from build123d import *

# Parameters (mm, degrees)
SKETCH1_R           = 1
BOSS_EXTRUDE1_DEPTH = 5
FILLET1_R           = 5
FILLET2_R           = 5
FILLET3_R           = 5
FILLET4_R           = 3


with BuildPart() as part:
    # Sketch1 → Boss-Extrude1 (new, symmetric)
    with BuildSketch(Plane(origin=(0, 0, 0), x_dir=(1, 0, 0), z_dir=(0, 1, 0))):
        Polygon((0, -60), (-14.281480067, -70), (-61.501480067, -70), (-99.58, -32.62), (-99.58, 0), (99.58, 0), (99.58, -32.62), (61.501480067, -70), (14.281480067, -70), align=None)
        with Locations(Location((96.58, -8.16, 0), (0, 0, 270))):
            Circle(SKETCH1_R, mode=Mode.SUBTRACT)
        with Locations(Location((96.58, -16.32, 0), (0, 0, 270))):
            Circle(SKETCH1_R, mode=Mode.SUBTRACT)
        with Locations(Location((96.58, -24.48, 0), (0, 0, 270))):
            Circle(SKETCH1_R, mode=Mode.SUBTRACT)
        with Locations(Location((-96.58, -24.48, 0), (0, 0, 90))):
            Circle(SKETCH1_R, mode=Mode.SUBTRACT)
        with Locations(Location((-96.58, -16.32, 0), (0, 0, 90))):
            Circle(SKETCH1_R, mode=Mode.SUBTRACT)
        with Locations(Location((-96.58, -8.16, 0), (0, 0, 90))):
            Circle(SKETCH1_R, mode=Mode.SUBTRACT)
    extrude(amount=BOSS_EXTRUDE1_DEPTH, both=True)

    # Fillet1
    fillet1_edges = [part.edges().sort_by_distance(p)[0] for p in [
        (-14.281480067, 0, 70),
        (14.281480067, 0, 70),
    ]]
    fillet(fillet1_edges, radius=FILLET1_R)

    # Fillet2
    fillet2_edges = [part.edges().sort_by_distance(p)[0] for p in [
        (-61.501480067, 0, 70),
        (61.501480067, 0, 70),
    ]]
    fillet(fillet2_edges, radius=FILLET2_R)

    # Fillet3
    fillet3_edges = [part.edges().sort_by_distance(p)[0] for p in [
        (-99.58, 0, 32.62),
        (99.58, 0, 32.62),
    ]]
    fillet(fillet3_edges, radius=FILLET3_R)

    # Fillet4
    fillet4_edges = [part.edges().sort_by_distance(p)[0] for p in [
        (-99.58, 0, 0),
        (99.58, 0, 0),
    ]]
    fillet(fillet4_edges, radius=FILLET4_R)

    # Fillet5
    # a fillet whose section is not a circle: 8 mm, written as the material it adds along each edge
    with BuildSketch(Plane(origin=(0, -5, 60), x_dir=(-0.8191520442889911, 0, 0.5735764363510473), z_dir=(0, 1, 0))) as fillet5_piece_1:
        with BuildLine():
            Bezier((5.601660306, 0), (0, 0), (-1.915880661, 5.263838853), weights=[1, 1, 1])
            Line((-1.915880661, 5.263838853), (0, 0))
            Line((0, 0), (5.601660306, 0))
        make_face()
    extrude(amount=10)


solid = part.part
Read the model definition and answer for the solid it produces. Units are mm, in the model's axes. Round coordinates to 2 decimals unless told otherwise and drop trailing zeros. Write each loop counter-clockwise with the first axis right and the second up, starting at its lowest first coordinate (ties: lowest second). Pieces come first, ordered by that corner, then holes.
Q1. Find section D-D on z = 54. Determine the outline of the cut face in (x, y), and give its area (3 significant figures).
Values:
outline: (-77.8, -5) - (77.8, -5) - (77.8, 5) - (-77.8, 5) - close
area: 1,560 mm2
Q2. The mould has two halves that part along X. Classify faces 1 (the face through (-8.731, 0.07, 66.113)), 2 (the face through (38, 0, 70)), 3 (the face through (80.767, 0.07, 51.088)), 4 (the face through (8.848, 0.07, 66.196)): released by +X, released by -X, zero draft, split by the parting line, or undercut.
Values:
face 1: undercut
face 2: zero draft
face 3: released by +X
face 4: undercut
Q3. Flat-ended cylindrical pins translate along their axes: P1, Ø2.5, axis at x = -96.58, z = 8.16, coming from the +Y side; P2, Ø2, axis at y = 3.5, z = 34, coming from the -X side; P3, Ø1.2, axis at x = 96.58, z = 16.32, coming from the +Y side. Find the tip coordinate at first contact, or state that the pin passes through.
Values:
P1: stops at y = 5
P2: stops at x = -98.92
P3: passes through
Q4. Find section A-A on z = 65.5. Determine the outline of the cut face in (x, y).
Values:
outline: (-66.09, -5) - (-7.85, -5) - (-7.85, 5) - (-66.09, 5) - close; (7.85, -5) - (66.09, -5) - (66.09, 5) - (7.85, 5) - close
Q5. Straight lines are drawn through the part: line 1 (X direction, y = 0, z = 8.16); line 2 (Z direction, x = -96.58, y = -1.75); line 3 (Z direction, x = -65.5, y = -3). For each, find the intervals that lie inside material, in ascending order.
Values:
line 1: x = -99.58 to -97.58, -95.58 to 95.58, 97.58 to 99.58
line 2: z = 0 to 7.16, 9.16 to 15.32, 17.32 to 23.48, 25.48 to 35.56
line 3: z = 0 to 66.07
Q6. Find section C-C on x = 86. Determine the outline of the cut face in (y, z).
Values:
outline: (-5, 0) - (5, 0) - (5, 45.95) - (-5, 45.95) - close
Q7. Find section B-B on y = 2. State how many separate pieces and enclosed holes the cut face has, and give its area (3 significant figures).
Values:
separate pieces: 1
enclosed holes: 6
area: 12,400 mm2
